The model under review builds one solid part; all positions refer to its coordinate system, in mm. A direction names the side the tool comes from. Coordinates: 2 decimals unless noted, no trailing zeros. Loops run counter-clockwise (first coordinate to the right, second up) from the corner with the lowest first, then second, coordinate; pieces in that order, holes last. Notation, with made-up numbers: M -28,-17.75 L 27,-17.75 A15 ccw 27,-6.75 Z; hole C -2.75,-40 d8. An arc over 180 degrees is marked long. One line per item, written item: value.
Autodesk Inventor part; units mm, degrees
ref_plane "YZ Plane" through (0, 0, 0) normal (1, 0, 0) x (0, 1, 0)
ref_plane "XZ Plane" through (0, 0, 0) normal (0, 1, 0) x (-1, 0, 0)
ref_plane "XY Plane" through (0, 0, 0) normal (0, 0, 1) x (1, 0, 0)
sketch "Эскиз1" plane through (0, 0, 0) normal (0, 1, 0) x (-1, 0, 0)
  circle A0 centre (0, 0) radius 22
  circle A1 centre (0, 0) radius 23.5
  circle A2 centre (0, 0) radius 26.5
  dimension "d0" = 44
  dimension "d1" = 47
  dimension "d2" = 53
extrude "Выдавливание1" add sketch "Эскиз1" along normal blind 12 contours A2
sketch "Эскиз2" plane through (0, 0, 0) normal (0, -1, 0) x (1, 0, 0)
  circle A0 centre (0, 0) radius 22
  circle A1 centre (0, 0) radius 23.5
  circle A2 centre (0, 0) radius 26.5
  dimension "d5" = 44
  dimension "d6" = 47
  dimension "d7" = 53
extrude "Выдавливание2" add sketch "Эскиз2" against normal blind 4 contours A1
sketch "Эскиз3" plane through (0, 0, 0) normal (0, -1, 0) x (1, 0, 0)
  circle A0 centre (0, 0) radius 22
  circle A1 centre (0, 0) radius 23.5
  circle A2 centre (0, 0) radius 26.5
  line L0 (-26.5, 26.5) -> (26.5, 26.5)
  line L1 (26.5, 26.5) -> (26.5, -26.5)
  line L2 (26.5, -26.5) -> (-26.5, -26.5)
  line L3 (-26.5, -26.5) -> (-26.5, 26.5)
  line L4 (-26.5, 26.5) -> (26.5, -26.5) construction
  line L5 (26.5, 26.5) -> (-26.5, -26.5) construction
  dimension "d10" = 44
  dimension "d11" = 47
  dimension "d12" = 53
  dimension "d13" = 53
  dimension "d14" = 53
extrude "Выдавливание3" add sketch "Эскиз3" against normal blind 4 contours L1 L2 A2 | A2 L0 L1 | A2 L3 L0 | L2 L3 A2
sketch "Эскиз4" plane through (0, 4, 0) normal (0, 1, 0) x (1, 0, 0)
  line L0 (0, 0) -> (21.2132, -21.2132)
  line L1 (0, 0) -> (30, 0) construction
  circle A0 centre (21.2132, -21.2132) radius 1.5
  dimension "d17" = 30
  dimension "d18" = 45
  dimension "d19" = 3
extrude "Выдавливание4" cut sketch "Эскиз4" against normal blind 4
pattern_circular "Круговой массив1" count 4 over 360 about axis through (0, -10, 0) along (0, 1, 0) of "Выдавливание4"
sketch "Эскиз5" plane through (0, 4, 0) normal (0, 1, 0) x (1, 0, 0)
  circle A0 centre (21.2132, -21.2132) radius 1.5
  circle A1 centre (21.2132, -21.2132) radius 3
  point P0 (0, 0)
  dimension "d25" = 6
extrude "Выдавливание5" cut sketch "Эскиз5" against normal blind 2
pattern_circular "Круговой массив2" count 4 over 360 about axis through (0, -10, 0) along (0, 1, 0) of "Выдавливание5"
fillet "Сопряжение1" radius 8.5 4 edges at (26.5, 2, -26.5) (26.5, 2, 26.5) (-26.5, 2, -26.5) (-26.5, 2, 26.5)
sketch "Эскиз6" plane through (0, 0, 0) normal (0, -1, 0) x (1, 0, 0)
  arc A0 (-18, 26.5) -> (-26.5, 18) centre (-18, 18) ccw
  line L0 (-26.5, -18) -> (-26.5, 18)
  arc A1 (-26.5, -18) -> (-18, -26.5) centre (-18, -18) ccw
  line L1 (18, -26.5) -> (-18, -26.5)
  arc A2 (18, -26.5) -> (26.5, -18) centre (18, -18) ccw
  line L2 (26.5, 18) -> (26.5, -18)
  arc A3 (26.5, 18) -> (18, 26.5) centre (18, 18) ccw
  line L3 (-18, 26.5) -> (18, 26.5)
  circle A4 centre (-21.2132, 21.2132) radius 1.5
  circle A5 centre (-21.2132, -21.2132) radius 1.5
  circle A6 centre (21.2132, -21.2132) radius 1.5
  circle A7 centre (21.2132, 21.2132) radius 1.5
  circle A8 centre (0, 0) radius 22
properties part number "000.001 - База лидара gjl gjlibgybr" material "Пластик АБС"
(1) Add section C-C on y = 8.25. State the section outline as (x, z) points.
Checks:
outline: C 0,0 d53; hole C 0,0 d47
(2) Add section A-A on x = -2. State the section outline as (y, z) points.
Checks:
outline: M 0,-26.5 L 4,-26.5 L 4,-26.42 L 12,-26.42 L 12,-23.41 L 4,-23.41 L 4,-21.91 L 0,-21.91 Z; M 0,21.91 L 4,21.91 L 4,23.41 L 12,23.41 L 12,26.42 L 4,26.42 L 4,26.5 L 0,26.5 Z
(3) Insertion check: pin 1 Ø5 at (x, z) = (-21.21, -21.21) entering from +Y; pin 2 Ø1.8 at (x, z) = (21.21, -21.21) entering from +Y; pin 3 Ø2 at (y, z) = (8.5, -7) entering from +X; pin 4 Ø2 at (x, y) = (-20.5, 2.5) entering from -Z. Each pin has a flat end and moves straight along its axis. Give the tip position at first contact, or say it passes through.
Checks:
pin 1: y = 2
pin 2: through
pin 3: x = 25.81
pin 4: z = -26.37
(4) Draft analysis for pull direction Z (two halves, no side actions). For faces 1 (the face through (-24.08, 2.03, 23.94)), 2 (the face through (-26.5, 2, 0)), 3 (the face through (0, 2, -26.5)), 4 (the face through (-22.4, 7.9, -7.1)), state which applies: pulls with the +Z half, pulls with the -Z half, needs draft (parallel to the pull), parting line crosses it, or undercut.
Checks:
face 1: pulls with the +Z half
face 2: needs draft
face 3: pulls with the -Z half
face 4: undercut
(5) Add section B-B on z = 14.5. State the section outline as (x, y) points, then the cut area to 3 significant figures.
Checks:
outline: M -26.5,0 L -16.55,0 L -16.55,4 L -18.49,4 L -18.49,12 L -22.18,12 L -22.18,4 L -26.5,4 Z; M 16.55,0 L 26.5,0 L 26.5,4 L 22.18,4 L 22.18,12 L 18.49,12 L 18.49,4 L 16.55,4 Z
area: 139 mm^2
(6) Tool access review of faces 5 (the face through (20, 4, 18)), 6 (the face through (-20, 4, -18)), 7 (the face through (23, 2, -23)), 8 (the face through (26.5, 2, 0)): name each direction out of +Z, -Z, +X, -X, +Y, -Y from which nothing blocks a thin tool from reaching the whole face with its end or side.
Checks:
face 5: +Z, +X, +Y
face 6: -Z, -X, +Y
face 7: +Y
face 8: +Z, -Z, +X, +Y, -Y
(7) To check wall thickness, follow L1, parallel to Z at x = 0, y = 10.75; L2, parallel to Y at x = 18.5, z = 21; L3, parallel to Z at x = -5.5, y = 11. State the ranges of each line that lie inside material, in increasing order. Write a range as [from, to].
Checks:
L1: [-26.5, -23.5], [23.5, 26.5]
L2: [0, 2]
L3: [-25.92, -22.85], [22.85, 25.92]
